Model file for the job. Use its own axes, mm. A direction names the side the tool comes from. Round coordinates to 2 decimals unless told otherwise and drop trailing zeros. Loops run counter-clockwise (first coordinate to the right, second up) from the corner with the lowest first, then second, coordinate; pieces in that order, holes last. Notation, with made-up numbers: (75, 52) - (112, 52) arc R24 ccw to (112, 82) - close; hole circle Ø2 at (33, 61). An arc over 180 degrees is marked (long way). Use one line per item in the form item = value.
from build123d import *

# Parameters (mm, degrees)
BOSS_EXTRUDE1_DEPTH = 2
FILLET1_R           = 1.5


with BuildPart() as part:
    # Sketch4 → Boss-Extrude1 (new body)
    with BuildSketch(Plane.XY):
        with BuildLine():
            Line((-13.050908111, 16), (-6.706499702, 16))
            Line((-6.706499702, 16), (3.293500298, 14.5))
            Line((3.293500298, 14.5), (17.050908111, 14.5))
            Line((17.050908111, 14.5), (17.050908111, 18))
            Line((17.050908111, 18), (23.550908111, 18))
            Line((23.550908111, 18), (23.550908111, 16))
            Line((23.550908111, 16), (21.550908111, 15))
            Line((21.550908111, 15), (21.550908111, 16))
            ThreePointArc((21.550908111, 16), (21.050908111, 16.5), (20.550908111, 16))
            Line((20.550908111, 16), (19.550908111, 16))
            ThreePointArc((19.550908111, 16), (19.050908111, 15.5), (19.550908111, 15))
            Line((19.550908111, 15), (19.550908111, 11.5))
            Line((19.550908111, 11.5), (18.050908111, 11.5))
            ThreePointArc((18.050908111, 11.5), (16.550908111, 10), (18.050908111, 8.5))
            Line((18.050908111, 8.5), (19.550908111, 8.5))
            Line((19.550908111, 8.5), (19.550908111, 5))
            ThreePointArc((19.550908111, 5), (19.050908111, 4.5), (19.550908111, 4))
            Line((19.550908111, 4), (20.550908111, 4))
            ThreePointArc((20.550908111, 4), (21.050908111, 3.5), (21.550908111, 4))
            Line((21.550908111, 4), (21.550908111, 5))
            Line((21.550908111, 5), (23.550908111, 4))
            Line((23.550908111, 4), (23.550908111, 2))
            Line((23.550908111, 2), (17.050908111, 2))
            Line((17.050908111, 2), (17.050908111, 5.5))
            Line((17.050908111, 5.5), (7.394672813, 5.5))
            ThreePointArc((7.394672813, 5.5), (1.329569341, 3.929982611), (-3.211963264, -0.38567682))
            Line((-3.211963264, -0.38567682), (-14.196296588, -18))
            Line((-14.196296588, -18), (-14.550908111, -18))
            ThreePointArc((-14.550908111, -18), (-15.300908111, -17.25), (-16.050908111, -18))
            Line((-16.050908111, -18), (-16.050908111, -19.5))
            ThreePointArc((-16.050908111, -19.5), (-16.197354721, -19.853553391), (-16.550908111, -20))
            Line((-16.550908111, -20), (-21.550908111, -20))
            ThreePointArc((-21.550908111, -20), (-21.904461502, -19.853553391), (-22.050908111, -19.5))
            Line((-22.050908111, -19.5), (-22.050908111, -18))
            ThreePointArc((-22.050908111, -18), (-22.300908111, -17.75), (-22.550908111, -18))
            Line((-22.550908111, -18), (-24.050908111, -18))
            Line((-24.050908111, -18), (-24.050908111, -14.588152482))
            ThreePointArc((-24.050908111, -14.588152482), (-23.749083006, -13.063848559), (-22.889156888, -11.769581233))
            ThreePointArc((-22.889156888, -11.769581233), (-20.39098235, -8.926642121), (-18.257237664, -5.800892224))
            ThreePointArc((-18.257237664, -5.800892224), (-16.93384188, 3.900322575), (-23.008225895, 11.579307131))
            ThreePointArc((-23.008225895, 11.579307131), (-23.770593485, 12.314190907), (-24.050908111, 13.335309027))
            Line((-24.050908111, 13.335309027), (-24.050908111, 14))
            Line((-24.050908111, 14), (-22.983920813, 14))
            ThreePointArc((-22.983920813, 14), (-22.421498589, 13.767037087), (-22.050908111, 14.25))
            Line((-22.050908111, 14.25), (-22.050908111, 15.5))
            ThreePointArc((-22.050908111, 15.5), (-21.904461502, 15.853553391), (-21.550908111, 16))
            Line((-21.550908111, 16), (-16.550908111, 16))
            ThreePointArc((-16.550908111, 16), (-16.197354721, 15.853553391), (-16.050908111, 15.5))
            Line((-16.050908111, 15.5), (-16.050908111, 14.25))
            ThreePointArc((-16.050908111, 14.25), (-15.680317634, 13.767037087), (-15.11789541, 14))
            Line((-15.11789541, 14), (-13.983920813, 14))
            ThreePointArc((-13.983920813, 14), (-13.421498589, 13.767037087), (-13.050908111, 14.25))
            Line((-13.050908111, 14.25), (-13.050908111, 16))
        make_face()
    extrude(amount=BOSS_EXTRUDE1_DEPTH)

    # Fillet1
    fillet1_edges = [part.edges().sort_by_distance(p)[0] for p in [
        (17.050908111, 14.5, 1),
        (17.050908111, 5.5, 1),
    ]]
    fillet(fillet1_edges, radius=FILLET1_R)


solid = part.part
1. Flat gauge pins, fed straight in: pin 1 (1.1 mm diameter, centred on y = 15.5, z = 0.5, fed in from -X); pin 2 (0.8 mm diameter, centred on x = 20, z = 1, fed in from -Y); pin 3 (0.6 mm diameter, centred on y = 3.5, z = 1, fed in from -X). Where does each tip first touch, or does it go through?
Geometry check:
pin_1 = -22.05
pin_2 = 2
pin_3 = -16.91
2. Tool access for faces 1 (the flat face through (19.551, 7, 1)), 2 (the cylindrical face through (16.62, 5.05, 1.01)), 3 (the flat face through (-13.051, 15, 1)), 4 (the flat face through (-23, -18, 1)): list every direction of +Z, -Z, +X, -X, +Y, -Y with a clear straight run to the whole face (end or side of a thin tool).
Geometry check:
face_1 = +Z, -Z, +X
face_2 = +Z, -Z, -Y
face_3 = +Z, -Z, +Y
face_4 = +Z, -Z, -X, -Y
3. Cut at A-A, the plane y = 4.5. Give the cut face in (x, z), plus the area to 3 significant figures.
Geometry check:
outline = (-17.11, 0) - (2.5, 0) - (2.5, 2) - (-17.11, 2) - close; (16.97, 0) - (19.05, 0) - (19.05, 2) - (16.97, 2) - close; (21.55, 0) - (22.55, 0) - (22.55, 2) - (21.55, 2) - close
area = 45.4 mm^2
4. Cut at B-B, the plane y = 10. Give the cut face in (x, z).
Geometry check:
outline = (-20.75, 0) - (16.55, 0) - (16.55, 2) - (-20.75, 2) - close
5. Wall check: probe 1 along Y at (x, z) = (18.5, 0.85); probe 2 along Y at (x, z) = (12, 0.9); probe 3 along Y at (x, z) = (-18.5, 1). Give the ranges that are in metal, low to high.
Geometry check:
probe_1 = 2 to 8.5, 11.5 to 18
probe_2 = 5.5 to 14.5
probe_3 = -20 to -6.2, 7.4 to 16
6. Pull direction Y, two halves, no side cores. Call faces 5 (the flat face through (-23.5, 14, 1)), 6 (the flat face through (21.551, 4.5, 1)), 7 (the flat face through (-24.051, -16, 1)): +Y half, -Y half, draft (parallel to the pull), parting line (faces both ways), or undercut.
Geometry check:
face_5 = +Y half
face_6 = undercut
face_7 = draft
7. Cut at C-C, the plane y = -4.5. Give the cut face in (x, z).
Geometry check:
outline = (-17.58, 0) - (-5.78, 0) - (-5.78, 2) - (-17.58, 2) - close
